Part print with two shaded views. Sizes in mm from the minimum x, y, z corner. A direction names the side the tool comes from. Give positions to 0.01 mm unless a question says otherwise; leave off trailing zeros. Return JSON: item names as keys, results as strings.
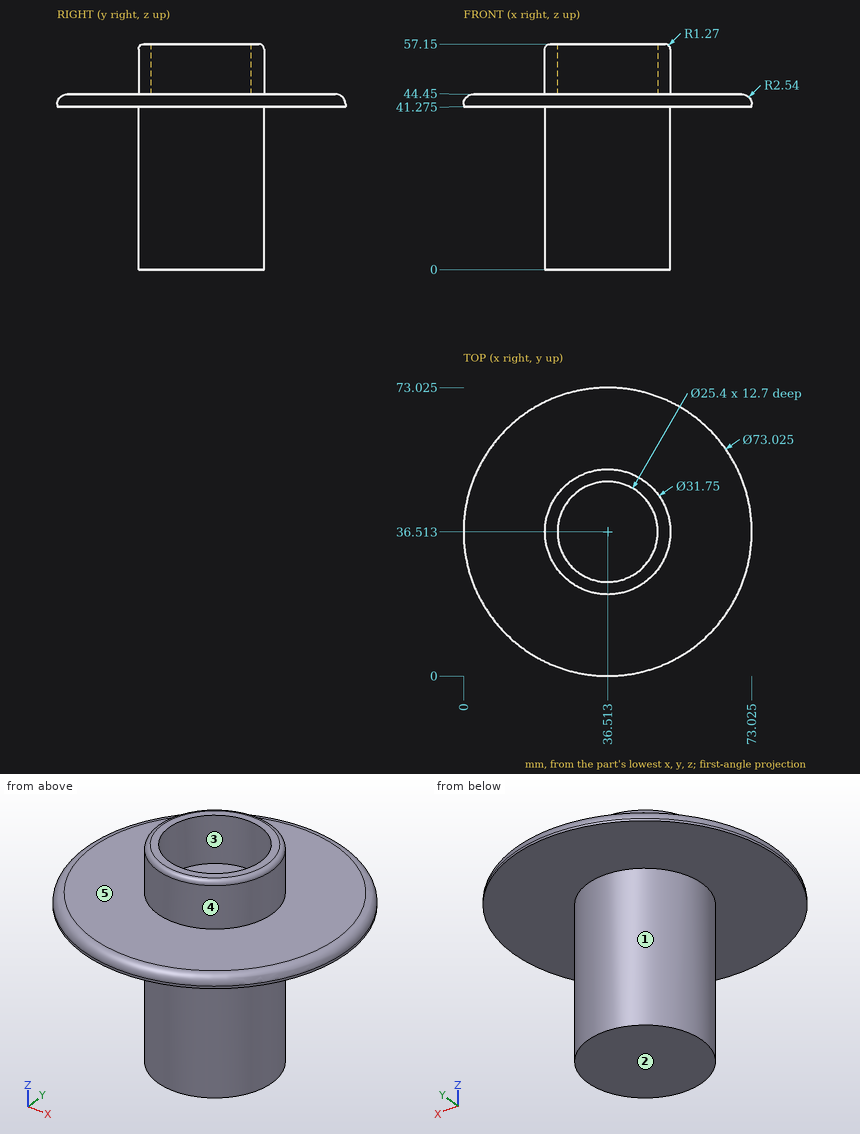
Q1. Pin check, flat tips, straight feed: pin 1 (8 mm diameter, centred on x = 46.5, y = 12.5, fed in from +Z); pin 2 (8 mm diameter, centred on y = 42, z = 21.5, fed in from -X); pin 3 (12 mm diameter, centred on x = 36, z = 16, fed in from -Y). Stop position of each tip, or through.
Established:
{"pin 1": "stops at z = 44.45", "pin 2": "stops at x = 20.71", "pin 3": "stops at y = 20.64"}
Q2. 3-axis set-ups, long thin cutter, end or side, ignore diameter. For the marked faces 1 and 2: which of +Z, -Z, +X, -X, +Y, -Y reach the whole face in a straight line?
Established:
{"face 1": "-Z", "face 2": "-Z, +X, -X, +Y, -Y"}
Q3. Probe line 1 along Z through (x, y) = (6, 21) (1 decimal); line 2 along X through (y, z) = (27, 53.5) (1 decimal); line 3 along Z through (x, y) = (22, 34.5). List the from-to ranges inside material, lowest first.
Established:
{"line 1": "z = 41.3 to 44.4", "line 2": "x = 23.8 to 28.1, 44.9 to 49.2", "line 3": "z = 0 to 57.15"}
Q4. Two-plate mould, pull along X, no slides. Class the marked faces 3, 4 and 5: +X half, -X half, draft (parallel to the pull), parting line (faces both ways), or undercut.
Established:
{"face 3": "undercut", "face 4": "parting line", "face 5": "draft"}
